```python
from build123d import *

# Parameters (mm, degrees)
BOSS_EXTRUDE1_DEPTH = 6.35
SKETCH2_W           = 406.4
SKETCH2_H           = 304.8
BOSS_EXTRUDE2_DEPTH = 161.925
SKETCH3_R           = 48.26
CUT_EXTRUDE1_DEPTH  = 161.925
SKETCH4_R           = 44.45
BOSS_EXTRUDE3_DEPTH = 38.1


with BuildPart() as part:
    # Sketch1 → Boss-Extrude1 (new body)
    with BuildSketch(Plane.XY):
        with BuildLine():
            Line((256.082305134, -169.999487802), (256.082305134, 169.999487802))
            ThreePointArc((256.082305134, 169.999487802), (257.049035071, 174.859567393), (259.802049013, 178.979743923))
            Line((259.802049013, 178.979743923), (322.888153673, 242.065848583))
            ThreePointArc((322.888153673, 242.065848583), (326.607897552, 251.046104704), (322.888153673, 260.026360825))
            Line((322.888153673, 260.026360825), (260.026360825, 322.888153673))
            ThreePointArc((260.026360825, 322.888153673), (251.046104704, 326.607897552), (242.065848583, 322.888153673))
            Line((242.065848583, 322.888153673), (180.680064074, 261.502369164))
            ThreePointArc((180.680064074, 261.502369164), (177.219980146, 260.814115678), (175.260000044, 263.747433194))
            Line((175.260000044, 263.747433194), (175.260000044, 279.4))
            ThreePointArc((175.260000044, 279.4), (120.65, 334.010000044), (66.039999956, 279.4))
            Line((66.039999956, 279.4), (66.039999956, 268.782305134))
            ThreePointArc((66.039999956, 268.782305134), (62.320256077, 259.802049013), (53.339999956, 256.082305134))
            Line((53.339999956, 256.082305134), (-53.339999956, 256.082305134))
            ThreePointArc((-53.339999956, 256.082305134), (-62.320256077, 259.802049013), (-66.039999956, 268.782305134))
            Line((-66.039999956, 268.782305134), (-66.039999956, 279.4))
            ThreePointArc((-66.039999956, 279.4), (-120.65, 334.010000044), (-175.260000044, 279.4))
            Line((-175.260000044, 279.4), (-175.260000044, 263.747433194))
            ThreePointArc((-175.260000044, 263.747433194), (-177.219980146, 260.814115678), (-180.680064074, 261.502369164))
            Line((-180.680064074, 261.502369164), (-242.065848583, 322.888153673))
            ThreePointArc((-242.065848583, 322.888153673), (-251.046104704, 326.607897552), (-260.026360825, 322.888153673))
            Line((-260.026360825, 322.888153673), (-322.888153673, 260.026360825))
            ThreePointArc((-322.888153673, 260.026360825), (-326.607897552, 251.046104704), (-322.888153673, 242.065848583))
            Line((-322.888153673, 242.065848583), (-259.802049013, 178.979743923))
            ThreePointArc((-259.802049013, 178.979743923), (-257.049035071, 174.859567393), (-256.082305134, 169.999487802))
            Line((-256.082305134, 169.999487802), (-256.082305134, -169.999487802))
            ThreePointArc((-256.082305134, -169.999487802), (-257.049035071, -174.859567393), (-259.802049013, -178.979743923))
            Line((-259.802049013, -178.979743923), (-322.888153673, -242.065848583))
            ThreePointArc((-322.888153673, -242.065848583), (-326.607897552, -251.046104704), (-322.888153673, -260.026360825))
            Line((-322.888153673, -260.026360825), (-260.026360825, -322.888153673))
            ThreePointArc((-260.026360825, -322.888153673), (-251.046104704, -326.607897552), (-242.065848583, -322.888153673))
            Line((-242.065848583, -322.888153673), (-180.680064074, -261.502369164))
            ThreePointArc((-180.680064074, -261.502369164), (-177.219980146, -260.814115678), (-175.260000044, -263.747433194))
            Line((-175.260000044, -263.747433194), (-175.260000044, -279.4))
            ThreePointArc((-175.260000044, -279.4), (-120.65, -334.010000044), (-66.039999956, -279.4))
            Line((-66.039999956, -279.4), (-66.039999956, -268.782305134))
            ThreePointArc((-66.039999956, -268.782305134), (-62.320256077, -259.802049013), (-53.339999956, -256.082305134))
            Line((-53.339999956, -256.082305134), (53.339999956, -256.082305134))
            ThreePointArc((53.339999956, -256.082305134), (62.320256077, -259.802049013), (66.039999956, -268.782305134))
            Line((66.039999956, -268.782305134), (66.039999956, -279.4))
            ThreePointArc((66.039999956, -279.4), (120.65, -334.010000044), (175.260000044, -279.4))
            Line((175.260000044, -279.4), (175.260000044, -263.747433194))
            ThreePointArc((175.260000044, -263.747433194), (177.219980146, -260.814115678), (180.680064074, -261.502369164))
            Line((180.680064074, -261.502369164), (242.065848583, -322.888153673))
            ThreePointArc((242.065848583, -322.888153673), (251.046104704, -326.607897552), (260.026360825, -322.888153673))
            Line((260.026360825, -322.888153673), (322.888153673, -260.026360825))
            ThreePointArc((322.888153673, -260.026360825), (326.607897552, -251.046104704), (322.888153673, -242.065848583))
            Line((322.888153673, -242.065848583), (259.802049013, -178.979743923))
            ThreePointArc((259.802049013, -178.979743923), (257.049035071, -174.859567393), (256.082305134, -169.999487802))
        make_face()
    extrude(amount=BOSS_EXTRUDE1_DEPTH)

    # Sketch2 → Boss-Extrude2 (add)
    with BuildSketch(Plane(origin=(0, 0, 0), x_dir=(-1, 0, 0), z_dir=(0, 0, -1))):
        Rectangle(SKETCH2_W, SKETCH2_H)
    extrude(amount=BOSS_EXTRUDE2_DEPTH)

    # Sketch3 → Cut-Extrude1 (cut)
    with BuildSketch(Plane(origin=(0, 0, 0), x_dir=(-1, 0, 0), z_dir=(0, 0, -1))):
        with Locations((120.65, 279.4)):
            Circle(SKETCH3_R)
        with Locations((-120.65, 279.4)):
            Circle(SKETCH3_R)
        with Locations((-120.65, -279.4)):
            Circle(SKETCH3_R)
        with Locations((120.65, -279.4)):
            Circle(SKETCH3_R)
    extrude(amount=-CUT_EXTRUDE1_DEPTH, mode=Mode.SUBTRACT)

    # Sketch4 → Boss-Extrude3 (add)
    with BuildSketch(Plane(origin=(203.2, 0, 0), x_dir=(0, 0, -1), z_dir=(1, 0, 0))):
        with Locations((80.9625, 101.6)):
            Circle(SKETCH4_R)
        with Locations((80.9625, -101.6)):
            Circle(SKETCH4_R)
    extrude(amount=BOSS_EXTRUDE3_DEPTH)


solid = part.part
```
Design review of the part built by this model. Coordinates are the model's own, in mm. A direction names the side the tool comes from. Give positions to 0.01 mm unless a question says otherwise; leave off trailing zeros. Write each loop counter-clockwise with the first axis right and the second up, starting at its lowest first coordinate (ties: lowest second). Pieces come first, ordered by that corner, then holes. Notation, with made-up numbers: (-36, -35) - (-22, -35) arc R6 ccw to (-22, -24) - close; hole circle Ø6 at (38, 30.25). An arc over 180 degrees is marked (long way). Return JSON: item names as keys, results as strings. Group by question number.
(1) We need section A-A, the plane x = 120.65. Give the boundary of the cut face in (y, z) (3 decimals), then the cut area to 3 significant figures.
(2) Machinability: for faces 1 (the flat face through (290.9, 210.08, 3.13)), 2 (the flat face through (-290.9, -210.08, 3.13)), 3 (the flat face through (3, -152.4, -80)), which of the approach directions +Z, -Z, +X, -X, +Y, -Y give a long, thin tool a straight path to every point of the face, cutting with its end or side? Answer none if there is none.
(3) Insertion check: pin 1 (3 mm diameter, centred on y = -274, z = 4.5, fed in from +X); pin 2 (10 mm diameter, centred on x = 82, z = -91.5, fed in from -Y); pin 3 (7 mm diameter, centred on y = 270.5, z = 4.5, fed in from -X). Each pin has a flat end and moves straight along its axis. Give the tip position at first contact, or say it passes through.
(4) We need section C-C, the plane x = -277. Give the boundary of the cut face in (y, z), then the cut area to 3 significant figures.
(5) We need section D-D, the plane z = -57.5. Give the boundary of the cut face in (x, y).
(6) To check wall thickness, follow probe 1 along Y at (x, z) = (-120, 5); probe 2 along X at (y, z) = (-279, 1); probe 3 along Y at (x, z) = (-201, -133). State the ranges of each line that lie inside material, in increasing order.
(7) Mouldability with a two-part tool opening along X and no side actions: class faces 4 (the flat face through (203.2, -2, -80)), 5 (the flat face through (-211.8, -292.62, 3.13)), 6 (the flat face through (-5, 5, 6.35)) as +X half, -X half, draft (parallel to the pull), parting line (faces both ways), or undercut.
Reported:
{
 "1": {"outline": "(-334.01, 0) - (-327.66, 0) - (-327.66, 6.35) - (-334.01, 6.35) - close; (-231.14, 0) - (-152.4, 0) - (-152.4, -161.925) - (152.4, -161.925) - (152.4, 0) - (231.14, 0) - (231.14, 6.35) - (-231.14, 6.35) - close; (327.66, 0) - (334.01, 0) - (334.01, 6.35) - (327.66, 6.35) - close", "area": "52,400 mm2"},
 "2": {"face 1": "+Z, -Z, +X", "face 2": "+Z, -Z, -X", "face 3": "-Z, +X, -X, -Y"},
 "3": {"pin 1": "stops at x = 310.41", "pin 2": "stops at y = -152.4", "pin 3": "stops at x = -315.91"},
 "4": {"outline": "(-305.91, 0) - (-196.18, 0) - (-196.18, 6.35) - (-305.91, 6.35) - close; (196.18, 0) - (305.91, 0) - (305.91, 6.35) - (196.18, 6.35) - close", "area": "1,390 mm2"},
 "5": {"outline": "(-203.2, -152.4) - (203.2, -152.4) - (203.2, -139.35) - (241.3, -139.35) - (241.3, -63.85) - (203.2, -63.85) - (203.2, 63.85) - (241.3, 63.85) - (241.3, 139.35) - (203.2, 139.35) - (203.2, 152.4) - (-203.2, 152.4) - close"},
 "6": {"probe 1": "y = -334.01 to -327.66, -231.14 to 231.14, 327.66 to 334.01", "probe 2": "x = -303.91 to -198.18, -175.26 to -168.91, -72.39 to -66.04, 66.04 to 72.39, 168.91 to 175.26, 198.18 to 303.91", "probe 3": "y = -152.4 to 152.4"},
 "7": {"face 4": "+X half", "face 5": "undercut", "face 6": "draft"}
}
